Part print with two shaded views. Sizes in mm from the minimum x, y, z corner. Coordinates: 2 decimals unless noted, no trailing zeros. Write each loop counter-clockwise with the first axis right and the second up, starting at its lowest first coordinate (ties: lowest second). Pieces come first, ordered by that corner, then holes.
Q1. Band-saw the part on B-B, the plane x = 12. Write the cut outline in (y, z).
Q2. Band-saw the part on A-A, the plane z = 32.5. Write the cut outline in (x, y).
Q3. Band-saw the part on C-C, the plane y = 2.15. State how many separate pieces and enclosed holes the cut face has, plus the area to 3 significant figures.
Q4. Drill centre lines: probe 1 along Z at (x, y) = (86, 1.6); probe 2 along X at (y, z) = (2.4, 9.5); probe 3 along X at (y, z) = (1.5, 53). Where is each one in solid material? Low to high.
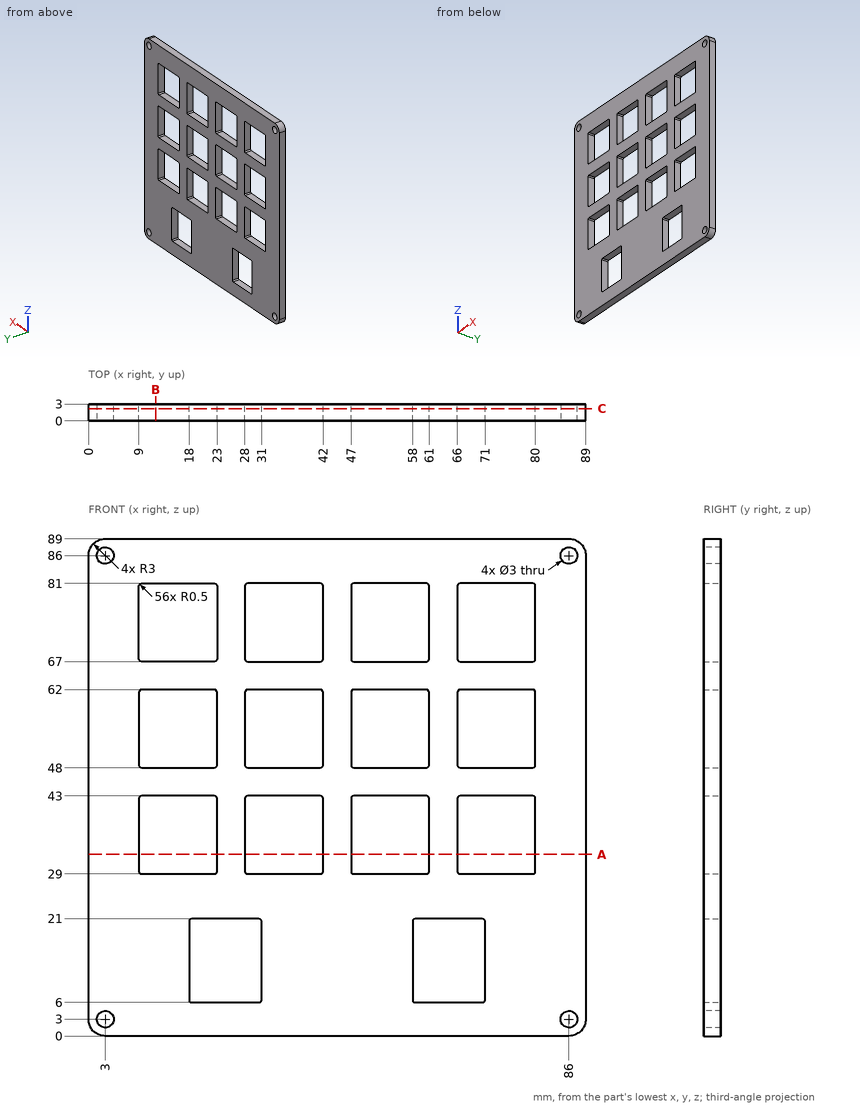
Answer sheet:
1. outline: (0, 0) - (3, 0) - (3, 29) - (0, 29) - close; (0, 43) - (3, 43) - (3, 48) - (0, 48) - close; (0, 62) - (3, 62) - (3, 67) - (0, 67) - close; (0, 81) - (3, 81) - (3, 89) - (0, 89) - close
2. outline: (0, 0) - (9, 0) - (9, 3) - (0, 3) - close; (23, 0) - (28, 0) - (28, 3) - (23, 3) - close; (42, 0) - (47, 0) - (47, 3) - (42, 3) - close; (61, 0) - (66, 0) - (66, 3) - (61, 3) - close; (80, 0) - (89, 0) - (89, 3) - (80, 3) - close
3. separate pieces: 1
3. enclosed holes: 18
3. area: 5,150 mm2
4. probe 1: z = 0 to 1.5, 4.5 to 84.5, 87.5 to 89
4. probe 2: x = 0 to 18, 31 to 58, 71 to 89
4. probe 3: x = 0 to 9, 23 to 28, 42 to 47, 61 to 66, 80 to 89
